Can you work these out from the model? Positions are in its coordinate system, mm. Face numbers are marked on the shaded views. Coordinates: 2 decimals unless noted, no trailing zeros. Order: outer loops, then holes, each group sorted by start corner. A loop starts at its lowest first (then second) coordinate and runs counter-clockwise, first axis right, second up. Notation, with made-up numbers: (8, 82.25) -> (21, 82.25) arc R4 ccw to (21, 87.25) -> close; hole circle Ø8 at (45.5, -22). An arc over 180 degrees is marked (long way). Write item = value, one per line. Start each with the question number.
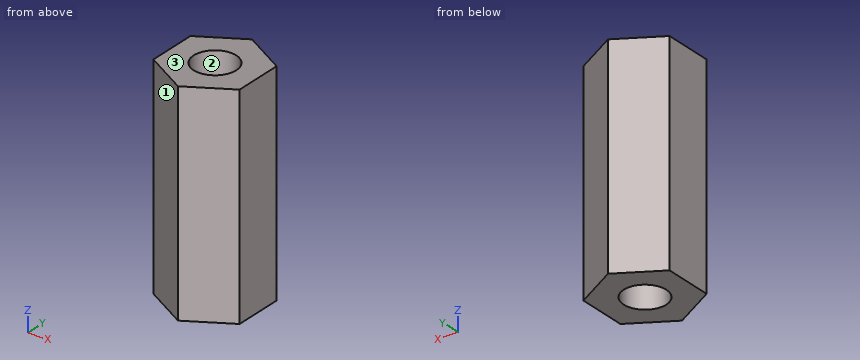
Autodesk Fusion 360 part; units mm, degrees
sketch "スケッチ1" plane through (0, 0, 0) normal (0, 0, 1) x (1, 0, 0)
  line L0 (3.5241, 6.0479) -> (-3.4756, 6.076)
  line L1 (-3.4756, 6.076) -> (-6.9997, 0.028)
  line L2 (-6.9997, 0.028) -> (-3.5241, -6.0479)
  line L3 (-3.5241, -6.0479) -> (3.4756, -6.076)
  line L4 (3.4756, -6.076) -> (6.9997, -0.028)
  line L5 (6.9997, -0.028) -> (3.5241, 6.0479)
  circle A0 centre (0, 0) radius 1.5
  line L6 (3.031, 1.7499) -> (0, 3.4999)
  line L7 (0, 3.4999) -> (-3.031, 1.7499)
  line L8 (-3.031, 1.7499) -> (-3.031, -1.7499)
  line L9 (-3.031, -1.7499) -> (0, -3.4999)
  line L10 (0, -3.4999) -> (3.031, -1.7499)
  line L11 (3.031, -1.7499) -> (3.031, 1.7499)
  dimension "d1" = 6.062
  dimension "d2" = 3
  dimension "d3" = 3.031
extrude "押し出し1" add sketch "スケッチ1" along normal blind 15 contours L6 L7 L8 L9 L10 L11
(1) Imagine slicing it at C-C (y = -0.75). Write out the boundary of the cut face in (x, z).
(2) Imagine slicing it at B-B (y = 0). Write out the boundary of the cut face in (x, z), plus the area to 3 significant figures.
(3) Imagine slicing it at D-D (x = 2.5). Write out the boundary of the cut face in (y, z), plus the area to 3 significant figures.
(4) Imagine slicing it at A-A (z = 2.5). Write out the boundary of the cut face in (x, y).
(5) Thinking about a two-plate mould opening in X: for the marked faces 1, 2 and 3, which applies, +X half, -X half, draft (parallel to the pull), parting line (faces both ways), or undercut?
(6) If I drill on L1, parallel to Y at x = 1.25, z = 1; L2, parallel to X at y = -0.75, z = 4.5; L3, parallel to Y at x = -1, z = 5.5, over which ranges is the centre line in solid material (lowest first)? Write a range as from..to.
(7) For P1, Ø2, axis at x = -1.5, z = 9.5, coming from the +Y side; P2, Ø1.5, axis at x = 1.5, z = 7.5, coming from the +Y side; P3, Ø3, axis at x = -1, z = 13, coming from the +Y side, each with a flat end and sliding along its axis, tell me the tip position at first contact or that it passes through.
Result set:
q1.outline = (-3.03, 0) -> (-1.3, 0) -> (-1.3, 15) -> (-3.03, 15) -> close; (1.3, 0) -> (3.03, 0) -> (3.03, 15) -> (1.3, 15) -> close
q2.outline = (-3.03, 0) -> (-1.5, 0) -> (-1.5, 15) -> (-3.03, 15) -> close; (1.5, 0) -> (3.03, 0) -> (3.03, 15) -> (1.5, 15) -> close
q2.area = 45.9 mm2
q3.outline = (-2.06, 0) -> (2.06, 0) -> (2.06, 15) -> (-2.06, 15) -> close
q3.area = 61.7 mm2
q4.outline = (-3.03, -1.75) -> (0, -3.5) -> (3.03, -1.75) -> (3.03, 1.75) -> (0, 3.5) -> (-3.03, 1.75) -> close; hole circle Ø3 at (0, 0)
q5.face_1 = -X half
q5.face_2 = undercut
q5.face_3 = draft
q6.L1 = -2.78..-0.83, 0.83..2.78
q6.L2 = -3.03..-1.3, 1.3..3.03
q6.L3 = -2.92..-1.12, 1.12..2.92
q7.P1 = 3.21
q7.P2 = 3.07
q7.P3 = 3.5
